Check sheet for the drawn part. Datum: minimum x, y, z corner. Units: mm. Round coordinates to 2 decimals unless told otherwise and drop trailing zeros. Write each loop counter-clockwise with the first axis right and the second up, starting at its lowest first coordinate (ties: lowest second). Pieces come first, ordered by that corner, then holes. Notation, with made-up numbers: M 25,10 L 53,10 A28 ccw 53,30 Z; hole C -0.75,9 d8. An arc over 180 degrees is marked long. Put each result on its own line as item: value.
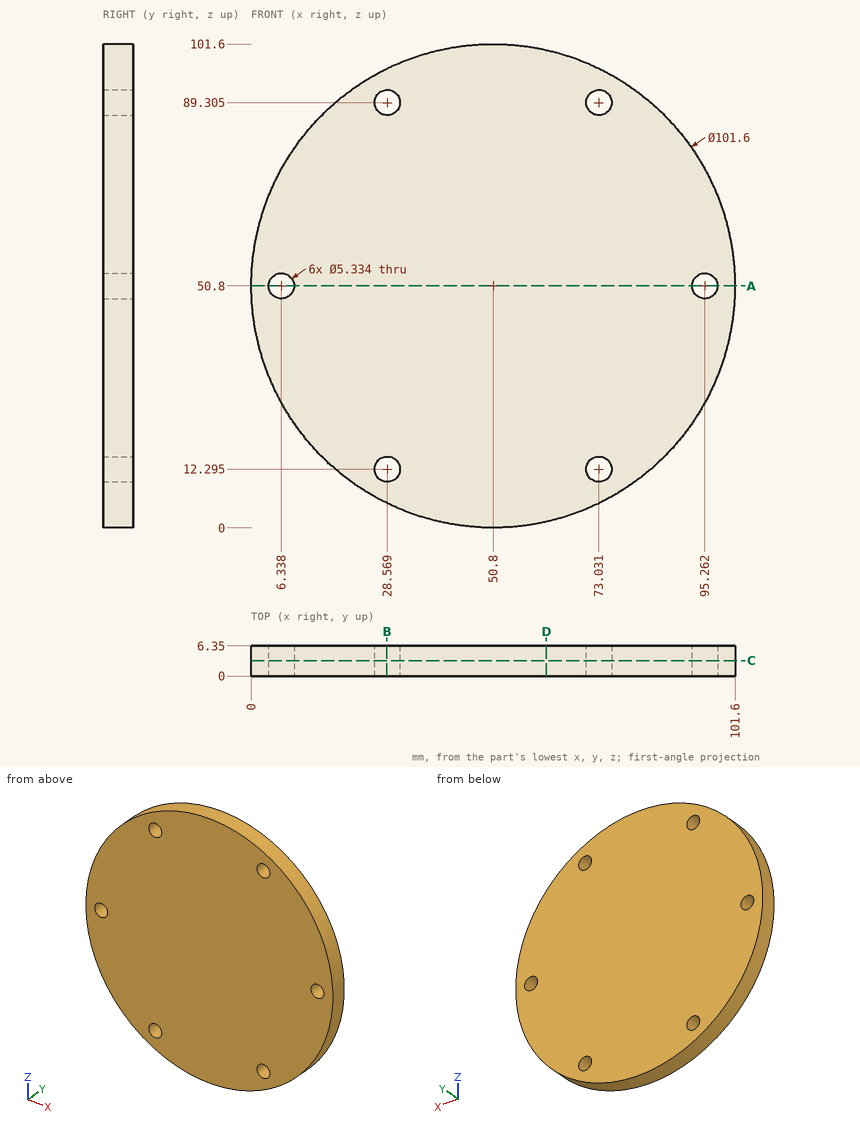
1. Cross-section at B-B (x = 28.5). Enter the section's corners in (y, z), then the cut area to 3 significant figures.
Computed values:
outline: M 0,5.16 L 6.35,5.16 L 6.35,9.63 L 0,9.63 Z; M 0,14.96 L 6.35,14.96 L 6.35,86.64 L 0,86.64 Z; M 0,91.97 L 6.35,91.97 L 6.35,96.44 L 0,96.44 Z
area: 512 mm2
2. Cross-section at C-C (y = 3.25). Enter the section's corners in (x, z) (1 decimal), then the cut area to 3 significant figures.
Computed values:
outline: C 50.8,50.8 d101.6; hole C 6.3,50.8 d5.3; hole C 28.6,12.3 d5.3; hole C 28.6,89.3 d5.3; hole C 73,12.3 d5.3; hole C 73,89.3 d5.3; hole C 95.3,50.8 d5.3
area: 7,970 mm2
3. Cross-section at A-A (z = 50.8). Enter the section's corners in (x, y) (3 decimals).
Computed values:
outline: M 0,0 L 3.671,0 L 3.671,6.35 L 0,6.35 Z; M 9.005,0 L 92.595,0 L 92.595,6.35 L 9.005,6.35 Z; M 97.929,0 L 101.6,0 L 101.6,6.35 L 97.929,6.35 Z
4. Depth check by flat-ended pin: pin 1 Ø3 at (y, z) = (5.5, 27) entering from -X; pin 2 Ø7 at (x, z) = (73.03, 89.31) entering from +Y; pin 3 Ø1.5 at (y, z) = (1, 45.5) entering from -X. Enter the tip coordinate at first touch or a pass-through.
Computed values:
pin 1: stops at x = 5.16
pin 2: stops at y = 6.35
pin 3: stops at x = 0.2
5. Cross-section at D-D (x = 62). Enter the section's corners in (y, z).
Computed values:
outline: M 0,1.25 L 6.35,1.25 L 6.35,100.35 L 0,100.35 Z
6. Scan lines: probe 1 along X at (y, z) = (2, 91.5) (1 decimal); probe 2 along X at (y, z) = (3.25, 52.5); probe 3 along Z at (x, y) = (76, 0.75). Record each from-to range of solid material in increasing order.
Computed values:
probe 1: x = 20.4 to 27.1, 30.1 to 71.5, 74.5 to 81.2
probe 2: x = 0.03 to 4.28, 8.39 to 93.21, 97.32 to 101.57
probe 3: z = 6.69 to 94.91
